Could you check a few things on this model? Use its own coordinates, in mm. A direction names the side the tool comes from. Coordinates: 2 decimals unless noted, no trailing zeros. Order: outer loops, then holes, each group sorted by start corner. A loop starts at its lowest first (then second) coordinate and runs counter-clockwise, first axis right, second up. Notation, with made-up numbers: (78.25, -37.5) - (105.25, -37.5) arc R17 cw to (105.25, -32.5) - close; hole circle Ø9 at (10.5, -3.75). An arc over 180 degrees is marked (long way). Answer as a JSON object with one key per item and string values. Group by question number.
(1) Imagine slicing it at B-B, the plane z = 0. Write out the boundary of the cut face in (x, y) (3 decimals).
(2) Imagine slicing it at D-D, the plane y = 1.7. Give the number of separate pieces and of enclosed holes in the cut face, and give its area (3 significant figures).
(3) Imagine slicing it at A-A, the plane z = 15.24. Write out the boundary of the cut face in (x, y) (3 decimals), and give its area (3 significant figures).
(4) Imagine slicing it at C-C, the plane x = -6. Write out the boundary of the cut face in (y, z) (3 decimals).
(5) Will these pins go through, and if not, where does the flat tip stop? P1, Ø1, axis at y = 1.5, z = -43, coming from the -X side; P2, Ø1, axis at x = 71, y = 1.5, coming from the -Z side (3 decimals); P3, Ø1, axis at x = -58.5, y = 2.5, coming from the +Z side (3 decimals).
(6) Please list where these lines run through material, in increasing order: probe 1 along X at (y, z) = (1, 15.24); probe 2 along Z at (x, y) = (-15.5, 2.7) (3 decimals); probe 3 along X at (y, z) = (0.4, -35.5) (1 decimal).
(7) We'd pull the mould along X, two halves only. Please class faces 6 (the flat face through (76.2, 2, 1)), 7 (the flat face through (73.025, 2, -36)), 8 (the flat face through (53, 2, 41.275)), 9 (the flat face through (-76.2, 2, 1)): pulls with the +X half, pulls with the -X half, needs draft (parallel to the pull), parting line crosses it, or undercut.
(8) Which directions (+Z, -Z, +X, -X, +Y, -Y) give clear straight access to the entire face, cutting with the end or side of a thin tool? Please do faces 1 (the flat face through (68.58, 2, -43)), 2 (the flat face through (53, 2, -41.275)), 3 (the flat face through (-30, 2, -41.275)), 4 (the flat face through (33, 2, 41.275)), 5 (the flat face through (-6, 2, -34.925)).
from build123d import *

# Parameters (mm, degrees)
SKETCH1_W                   = 10.16
SKETCH1_H                   = 3.175
SKETCH1_W_2                 = 152.4
SKETCH1_H_2                 = 82.55
SKETCH1_R                   = 7.747
BOSS_EXTRUDE1_DEPTH         = 3.175
SKETCH2_R                   = 2.06375
CASTER_MOUNTING_HOLES_DEPTH = 89.274136218
SKETCH3_W                   = 4.7625
SKETCH3_H                   = 3.175
CUT_EXTRUDE1_DEPTH          = 89.274136218
LPATTERN1_COUNT             = 2
LPATTERN1_PITCH             = 76.2
LPATTERN1_COUNT_DIR2        = 2
LPATTERN1_PITCH_DIR2        = 73.025


with BuildPart() as part:
    # Sketch1 → Boss-Extrude1 (new body)
    # profile 1 of 7: a face of its own
    with BuildSketch(Plane(origin=(0, 0, 0), x_dir=(1, 0, 0), z_dir=(0, 1, 0))):
        with Locations((43.18, -42.8625)):
            Rectangle(SKETCH1_W, SKETCH1_H)
    # profile 2 of 7: a face of its own
    with BuildSketch(Plane(origin=(0, 0, 0), x_dir=(1, 0, 0), z_dir=(0, 1, 0))):
        Rectangle(SKETCH1_W_2, SKETCH1_H_2)
        with Locations(Location((-65.076590574, 0, 0), (0, 0, 270))):
            Circle(SKETCH1_R, mode=Mode.SUBTRACT)
    # profile 3 of 7: a face of its own
    with BuildSketch(Plane(origin=(0, 0, 0), x_dir=(1, 0, 0), z_dir=(0, 1, 0))):
        with Locations((63.5, -42.8625)):
            Rectangle(SKETCH1_W, SKETCH1_H)
    # profile 4 of 7: a face of its own
    with BuildSketch(Plane(origin=(0, 0, 0), x_dir=(1, 0, 0), z_dir=(0, 1, 0))):
        with Locations((22.86, -42.8625)):
            Rectangle(SKETCH1_W, SKETCH1_H)
    # profile 5 of 7: a face of its own
    with BuildSketch(Plane(origin=(0, 0, 0), x_dir=(1, 0, 0), z_dir=(0, 1, 0))):
        with Locations((63.5, 42.8625)):
            Rectangle(SKETCH1_W, SKETCH1_H)
    # profile 6 of 7: a face of its own
    with BuildSketch(Plane(origin=(0, 0, 0), x_dir=(1, 0, 0), z_dir=(0, 1, 0))):
        with Locations((43.18, 42.8625)):
            Rectangle(SKETCH1_W, SKETCH1_H)
    # profile 7 of 7: a face of its own
    with BuildSketch(Plane(origin=(0, 0, 0), x_dir=(1, 0, 0), z_dir=(0, 1, 0))):
        with Locations((22.86, 42.8625)):
            Rectangle(SKETCH1_W, SKETCH1_H)
    extrude(amount=BOSS_EXTRUDE1_DEPTH)

    # Sketch2 → Caster Mounting Holes (cut, through all)
    with BuildSketch(Plane(origin=(0, 3.175, 0), x_dir=(1, 0, 0), z_dir=(0, 1, 0))):
        with Locations(Location((-47.3754273, 15.24, 0), (0, 0, 270))):
            Circle(SKETCH2_R)
        with Locations(Location((-22.9914273, 15.24, 0), (0, 0, 270))):
            Circle(SKETCH2_R)
        with Locations(Location((-22.9914273, -15.24, 0), (0, 0, 270))):
            Circle(SKETCH2_R)
        with Locations(Location((-47.3754273, -15.24, 0), (0, 0, 270))):
            Circle(SKETCH2_R)
    extrude(amount=-CASTER_MOUNTING_HOLES_DEPTH, mode=Mode.SUBTRACT)

    # Sketch3 → Cut-Extrude1 (cut, through all)
    with BuildSketch(Plane(origin=(0, 3.175, 0), x_dir=(1, 0, 0), z_dir=(0, 1, 0))):
        with Locations((62.70625, 36.5125)):
            Rectangle(SKETCH3_W, SKETCH3_H)
        with Locations((70.64375, 36.5125)):
            Rectangle(SKETCH3_W, SKETCH3_H)
    cut_extrude1 = extrude(amount=-CUT_EXTRUDE1_DEPTH, mode=Mode.SUBTRACT)

    # LPattern1: Cut-Extrude1 2 × 2
    with Locations(*[(-i * LPATTERN1_PITCH, 0, j * LPATTERN1_PITCH_DIR2) for i in range(LPATTERN1_COUNT) for j in range(LPATTERN1_COUNT_DIR2) if (i, j) != (0, 0)]):
        add(cut_extrude1, mode=Mode.SUBTRACT)


solid = part.part
Result set:
{
 "1": {"outline": "(-76.2, 0) - (-72.824, 0) - (-72.824, 3.175) - (-76.2, 3.175) - close; (-57.33, 0) - (76.2, 0) - (76.2, 3.175) - (-57.33, 3.175) - close"},
 "2": {"separate pieces": "1", "enclosed holes": "13", "area": "12,400 mm^2"},
 "3": {"outline": "(-76.2, 0) - (-49.439, 0) - (-49.439, 3.175) - (-76.2, 3.175) - close; (-45.312, 0) - (-25.055, 0) - (-25.055, 3.175) - (-45.312, 3.175) - close; (-20.928, 0) - (76.2, 0) - (76.2, 3.175) - (-20.928, 3.175) - close", "area": "458 mm^2"},
 "4": {"outline": "(0, -41.275) - (3.175, -41.275) - (3.175, -38.1) - (0, -38.1) - close; (0, -34.925) - (3.175, -34.925) - (3.175, 34.925) - (0, 34.925) - close; (0, 38.1) - (3.175, 38.1) - (3.175, 41.275) - (0, 41.275) - close"},
 "5": {"P1": "stops at x = 17.78", "P2": "stops at z = -41.275", "P3": "stops at z = 41.275"},
 "6": {"probe 1": "x = -76.2 to -49.44, -45.31 to -25.06, -20.93 to 76.2", "probe 2": "z = -41.275 to -38.1, -34.925 to 34.925, 38.1 to 41.275", "probe 3": "x = -76.2 to -15.9, -11.1 to -7.9, -3.2 to 60.3, 65.1 to 68.3, 73 to 76.2"},
 "7": {"face 6": "pulls with the +X half", "face 7": "undercut", "face 8": "undercut", "face 9": "pulls with the -X half"},
 "8": {"face 1": "-Z, +X, +Y, -Y", "face 2": "-Z, +Y, -Y", "face 3": "-Z, -X, +Y, -Y", "face 4": "+Z, +Y, -Y", "face 5": "+Y, -Y"}
}
